Print and shaded views of the part. All mm, measured from the part's lowest x, y and z. Round coordinates to 2 decimals unless told otherwise and drop trailing zeros. Order: outer loops, then holes, each group sorted by start corner. A loop starts at its lowest first (then second) coordinate and runs counter-clockwise, first axis right, second up. Notation, with made-up numbers: (82, -12.75) -> (135, -12.75) arc R19 cw to (135, 10.25) -> close; hole circle Ø5 at (52.5, 59). An arc over 180 degrees is marked (long way). Answer as CSV lines item,"result".
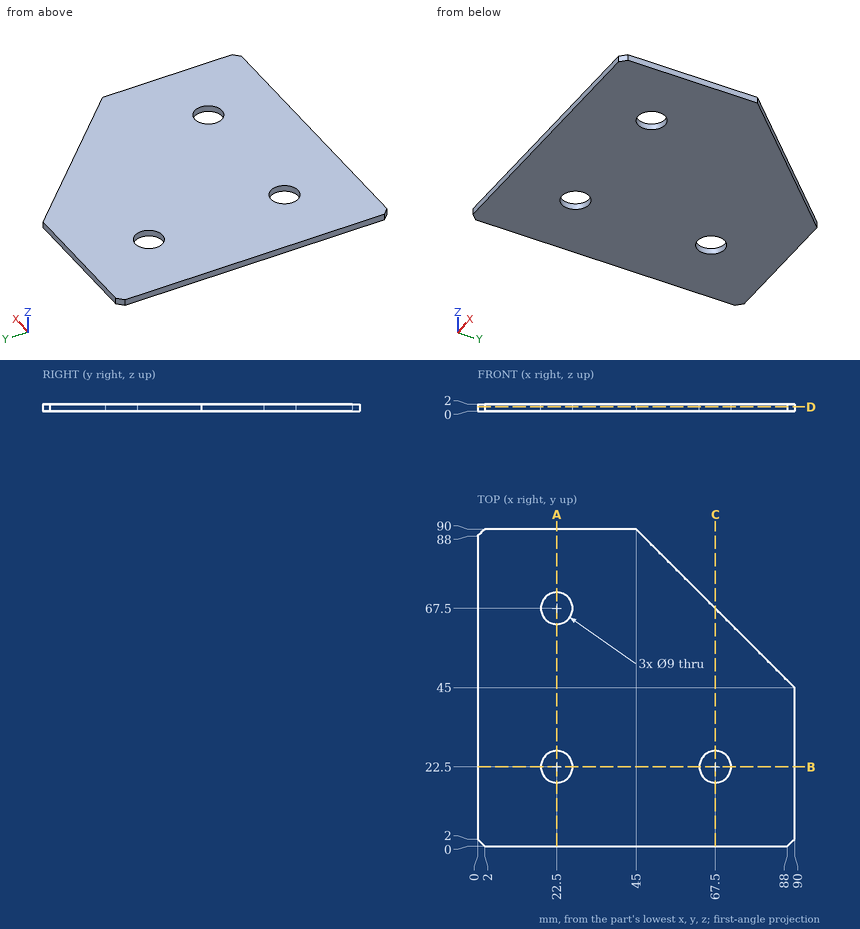
Q1. Saw through at C-C (x = 67.5). Write the cut outline in (y, z).
Checks:
outline,"(0, 0) -> (18, 0) -> (18, 2) -> (0, 2) -> close; (27, 0) -> (67.5, 0) -> (67.5, 2) -> (27, 2) -> close"
Q2. Saw through at D-D (z = 1.2). Write the cut outline in (x, y).
Checks:
outline,"(0, 2) -> (2, 0) -> (88, 0) -> (90, 2) -> (90, 45) -> (45, 90) -> (2, 90) -> (0, 88) -> close; hole circle Ø9 at (22.5, 22.5); hole circle Ø9 at (22.5, 67.5); hole circle Ø9 at (67.5, 22.5)"
Q3. Wall check: L1, parallel to Y at x = 22.5, z = 0.65; L2, parallel to Y at x = 26, z = 1.95. Give the ranges that are in metal, low to high. Write a range as [from, to].
Checks:
L1,"[0, 18], [27, 63], [72, 90]"
L2,"[0, 19.67], [25.33, 64.67], [70.33, 90]"
Q4. Saw through at A-A (x = 22.5). Write the cut outline in (y, z).
Checks:
outline,"(0, 0) -> (18, 0) -> (18, 2) -> (0, 2) -> close; (27, 0) -> (63, 0) -> (63, 2) -> (27, 2) -> close; (72, 0) -> (90, 0) -> (90, 2) -> (72, 2) -> close"
